from build123d import *

# Parameters (mm, degrees)
SKETCH1_W           = 65
SKETCH1_H           = 46
SKETCH1_R           = 4.6
SKETCH1_R_2         = 2.5
BOSS_EXTRUDE1_DEPTH = 5
SKETCH2_R           = 1.6
CUT_EXTRUDE1_DEPTH  = 10
SKETCH3_W           = 4
SKETCH3_H           = 46
CUT_EXTRUDE2_DEPTH  = 6
SKETCH4_W           = 6
SKETCH4_H           = 46
BOSS_EXTRUDE2_DEPTH = 5
FILLET1_R           = 10
FILLET2_R           = 1


with BuildPart() as part:
    # Sketch1 → Boss-Extrude1 (new body)
    with BuildSketch(Plane.XY):
        with Locations((7.5, 0)):
            Rectangle(SKETCH1_W, SKETCH1_H)
        Circle(SKETCH1_R, mode=Mode.SUBTRACT)
        with Locations((30, -18.25)):
            Circle(SKETCH1_R_2, mode=Mode.SUBTRACT)
        with BuildLine():
            ThreePointArc((39.5, 0), (23.282485579, -6.717514421), (30, 9.5))
            ThreePointArc((30, 9.5), (36.717514421, 6.717514421), (39.5, 0))
        make_face(mode=Mode.SUBTRACT)
        with BuildLine():
            ThreePointArc((32.5, 18.25), (31.767766953, 16.482233047), (30, 15.75))
            ThreePointArc((30, 15.75), (28.232233047, 20.017766953), (32.5, 18.25))
        make_face(mode=Mode.SUBTRACT)
    extrude(amount=BOSS_EXTRUDE1_DEPTH)

    # Sketch2 → Cut-Extrude1 (cut)
    with BuildSketch(Plane.XY.offset(5)):
        with Locations((7, 19)):
            Circle(SKETCH2_R)
        with Locations((-5, -19)):
            Circle(SKETCH2_R)
        with Locations((-17, 19)):
            Circle(SKETCH2_R)
        with Locations((-5, 19)):
            Circle(SKETCH2_R)
        with Locations((7, -19)):
            Circle(SKETCH2_R)
        with Locations((-17, -19)):
            Circle(SKETCH2_R)
    extrude(amount=-CUT_EXTRUDE1_DEPTH, mode=Mode.SUBTRACT)

    # Sketch3 → Cut-Extrude2 (cut, through all)
    with BuildSketch(Plane.XY.offset(5)):
        with Locations((-23, 0)):
            Rectangle(SKETCH3_W, SKETCH3_H)
    extrude(amount=-CUT_EXTRUDE2_DEPTH, mode=Mode.SUBTRACT)

    # Sketch4 → Boss-Extrude2 (add)
    with BuildSketch(Plane.XY.offset(5)):
        with Locations((43, 0)):
            Rectangle(SKETCH4_W, SKETCH4_H)
    extrude(amount=-BOSS_EXTRUDE2_DEPTH)

    # Fillet1
    fillet1_edges = [part.edges().sort_by_distance(p)[0] for p in [
        (46, -23, 2.5),
        (46, 23, 2.5),
    ]]
    fillet(fillet1_edges, radius=FILLET1_R)

    # Fillet2
    fillet2_edges = [part.edges().sort_by_distance(p)[0] for p in [
        (-21, 23, 2.5),
        (-21, -23, 2.5),
    ]]
    fillet(fillet2_edges, radius=FILLET2_R)


solid = part.part
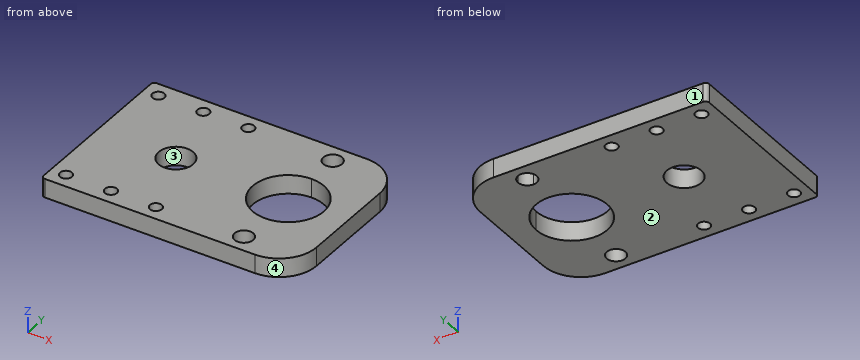
Build history of the part. All positions in model axes, mm. Face numbers are marked on the shaded views. Coordinates: 2 decimals unless noted, no trailing zeros. Write each loop counter-clockwise with the first axis right and the second up, starting at its lowest first coordinate (ties: lowest second). Pieces come first, ordered by that corner, then holes.
(1) Cut at A-A on z = 2.85. State how many separate pieces and enclosed holes the cut face has, and give its area (3 significant figures).
(2) Cut at C-C on y = 8. List the corners of the cut face in (x, z).
(3) Mould opens along Y. For the marked faces 1, 2, 3 and 4 say: pulls with the +Y half, pulls with the -Y half, needs draft (parallel to the pull), parting line crosses it, or undercut.
(4) Drill centre lines: line 1 (Y direction, x = 30, z = 3.65); line 2 (X direction, y = 3.5, z = 3.4); line 3 (X direction, y = 18, z = 2.65). Where is each one in solid material? Low to high.
(5) Cut at B-B on x = -17. List the corners of the cut face in (y, z), and give its area (3 significant figures).
(6) Cut at D-D on y = -3.5. List the corners of the cut face in (x, z).
Working result:
1. separate pieces: 1
1. enclosed holes: 10
1. area: 2,600 mm2
2. outline: (-21, 0) - (24.88, 0) - (24.88, 5) - (-21, 5) - close; (35.12, 0) - (46, 0) - (46, 5) - (35.12, 5) - close
3. face 1: pulls with the +Y half
3. face 2: needs draft
3. face 3: undercut
3. face 4: pulls with the -Y half
4. line 1: y = -23 to -20.75, -15.75 to -9.5, 9.5 to 15.75, 20.75 to 23
4. line 2: x = -21 to -2.98, 2.98 to 21.17, 38.83 to 46
4. line 3: x = -21 to -18.25, -15.75 to -6.25, -3.75 to 5.75, 8.25 to 27.51, 32.49 to 44.66
5. outline: (-23, 0) - (-20.6, 0) - (-20.6, 5) - (-23, 5) - close; (-17.4, 0) - (17.4, 0) - (17.4, 5) - (-17.4, 5) - close; (20.6, 0) - (23, 0) - (23, 5) - (20.6, 5) - close
5. area: 198 mm2
6. outline: (-21, 0) - (-2.98, 0) - (-2.98, 5) - (-21, 5) - close; (2.98, 0) - (21.17, 0) - (21.17, 5) - (2.98, 5) - close; (38.83, 0) - (46, 0) - (46, 5) - (38.83, 5) - close
